Verification items for this drawing (mm, ordinates from the low corner). Give positions to 0.01 mm unless a question says otherwise; leave off trailing zeros. Write each loop counter-clockwise with the first axis right and the second up, starting at its lowest first coordinate (ties: lowest second). Pieces come first, ordered by that corner, then holes. Notation, with made-up numbers: M 57,30.5 L 115,30.5 A21 ccw 115,45.5 Z; hole C 4,35 d9. An arc over 180 degrees is marked long. Write each question's results on one line, items separated by ' | '.
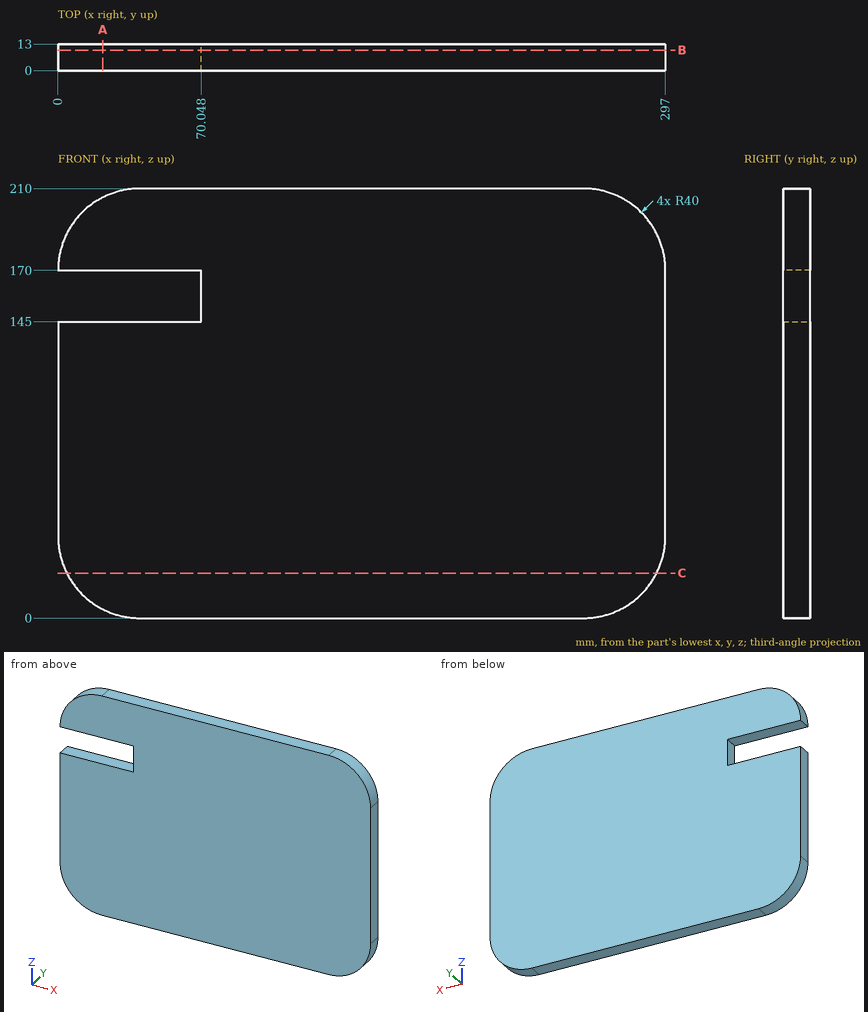
Q1. Section check A-A (x = 22). Enter the section's corners in (y, z).
Answer key:
outline: M 0,4.28 L 13,4.28 L 13,145 L 0,145 Z; M 0,170 L 13,170 L 13,205.72 L 0,205.72 Z
Q2. Section check B-B (y = 10). Enter the section's corners in (x, z).
Answer key:
outline: M 0,40 A40 ccw 40,0 L 257,0 A40 ccw 297,40 L 297,170 A40 ccw 257,210 L 40,210 A40 ccw 0,170 L 70.05,170 L 70.05,145 L 0,145 Z
Q3. Material ranges on probe 1 along Z at (x, y) = (61.5, 7); probe 2 along X at (y, z) = (11, 146.5); probe 3 along Z at (x, y) = (15, 5.75) (1 decimal), recorded low to high. Write a range as [from, to].
Answer key:
probe 1: z = [0, 145], [170, 210] | probe 2: x = [70.05, 297] | probe 3: z = [8.8, 145], [170, 201.2]
Q4. Depth check by flat-ended pin: P1, Ø4, axis at x = 38, y = 4.5, coming from the +Z side; P2, Ø6.5, axis at y = 6, z = 162, coming from the -X side. Enter the tip coordinate at first touch or a pass-through.
Answer key:
P1: stops at z = 210 | P2: stops at x = 70.05
Q5. Section check C-C (z = 22). Enter the section's corners in (x, y), then the cut area to 3 significant figures.
Answer key:
outline: M 4.28,0 L 292.72,0 L 292.72,13 L 4.28,13 Z | area: 3,750 mm2
